Model file for the job. Use its own axes, mm. Face numbers are marked on the shaded views. A direction names the side the tool comes from. Round coordinates to 2 decimals unless told otherwise and drop trailing zeros. Write each loop counter-clockwise with the first axis right and the second up, starting at its lowest first coordinate (ties: lowest second). Pieces come first, ordered by that corner, then holes. Notation, with made-up numbers: (-23, 60) - (-19, 60) arc R11 cw to (-19, 67) - close; hole circle Ø7 at (79, 35). An arc over 180 degrees is marked (long way). One line per item, written item: value.
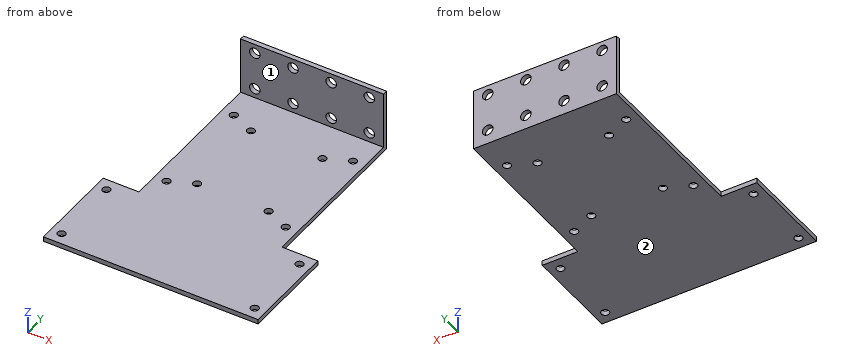
from build123d import *

# Parameters (mm, degrees)
F0_W     = 90
F0_H     = 110
F1_DEPTH = 26
F2_W     = 108
F2_H     = 24
F3_DEPTH = 90.001
F5_D     = 4.4
F6_W     = 15
F6_H     = 70
F7_DEPTH = 26.001
F9_D     = 3.3


with BuildPart() as f1:
    # F0 (on Top) → F1 (new body)
    with BuildSketch(Plane.XY):
        Rectangle(F0_W, F0_H)
    extrude(amount=F1_DEPTH)

    # F2 (on face) → F3 (cut, through all)
    with BuildSketch(Plane.YZ.offset(45)):
        with Locations((-1, 14)):
            Rectangle(F2_W, F2_H)
    extrude(amount=-F3_DEPTH, mode=Mode.SUBTRACT)

    # F5 (through all)
    with Locations(Plane(origin=(0, 55, 0), x_dir=(-1, 0, 0), z_dir=(0, 1, 0))):
        with Locations((-8, 22), (8, 22), (8, 6), (-8, 6), (-24, 22), (24, 22), (24, 6), (-24, 6)):
            Hole(F5_D / 2)

    # F6 (on face) → F7 (cut, through all)
    with BuildSketch(Plane(origin=(0, 0, 0), x_dir=(1, 0, 0), z_dir=(0, 0, -1))):
        with Locations((-37.5, -20)):
            Rectangle(F6_W, F6_H)
        with Locations((37.5, -20)):
            Rectangle(F6_W, F6_H)
    extrude(amount=-F7_DEPTH, mode=Mode.SUBTRACT)

    # F9 (through all)
    with Locations(Plane.XY.offset(2)):
        with Locations((25, 40.5), (15, 36), (-15, 36), (-25, 40.5), (-25, -4.5), (-15, 0), (15, 0), (25, -4.5), (40.5, -20), (40.5, -50), (-40.5, -50), (-40.5, -20)):
            Hole(F9_D / 2)


solid = f1.part
1. Wall check: probe 1 along Z at (x, y) = (8, 53.8); probe 2 along Z at (x, y) = (19, -42.5); probe 3 along Y at (x, z) = (10, 23.75). Give the ranges that are in metal, low to high. Write a range as [from, to].
Report:
probe 1: [0, 3.8], [8.2, 19.8], [24.2, 26]
probe 2: [0, 2]
probe 3: [53, 55]
2. Band-saw the part on A-A on y = 36. Write the cut outline in (x, z).
Report:
outline: (-30, 0) - (-16.65, 0) - (-16.65, 2) - (-30, 2) - close; (-13.35, 0) - (13.35, 0) - (13.35, 2) - (-13.35, 2) - close; (16.65, 0) - (30, 0) - (30, 2) - (16.65, 2) - close
3. Band-saw the part on B-B on x = 15. Write the cut outline in (y, z), plus the area to 3 significant figures.
Report:
outline: (-55, 0) - (-1.65, 0) - (-1.65, 2) - (-55, 2) - close; (1.65, 0) - (34.35, 0) - (34.35, 2) - (1.65, 2) - close; (37.65, 0) - (55, 0) - (55, 26) - (53, 26) - (53, 2) - (37.65, 2) - close
area: 255 mm²
4. Band-saw the part on D-D on x = -40.5. Write the cut outline in (y, z), plus the area to 3 significant figures.
Report:
outline: (-55, 0) - (-51.65, 0) - (-51.65, 2) - (-55, 2) - close; (-48.35, 0) - (-21.65, 0) - (-21.65, 2) - (-48.35, 2) - close; (-18.35, 0) - (-15, 0) - (-15, 2) - (-18.35, 2) - close
area: 66.8 mm²
5. Tool access for the marked faces 1 and 2: list every direction of +Z, -Z, +X, -X, +Y, -Y with a clear straight run to the whole face (end or side of a thin tool).
Report:
face 1: +Z, +X, -X, -Y
face 2: -Z, +X, -X, +Y, -Y
6. Band-saw the part on C-C on x = -25. Write the cut outline in (y, z).
Report:
outline: (-55, 0) - (-6.15, 0) - (-6.15, 2) - (-55, 2) - close; (-2.85, 0) - (38.85, 0) - (38.85, 2) - (-2.85, 2) - close; (42.15, 0) - (55, 0) - (55, 4.04) - (53, 4.04) - (53, 2) - (42.15, 2) - close; (53, 7.96) - (55, 7.96) - (55, 20.04) - (53, 20.04) - close; (53, 23.96) - (55, 23.96) - (55, 26) - (53, 26) - close
7. Drop flat-ended pins along their axis: pin 1 (2 mm diameter, centred on x = -1.5, z = 7, fed in from -Y); pin 2 (3.5 mm diameter, centred on x = 8, z = 6, fed in from +Y); pin 3 (4.5 mm diameter, centred on x = -25, y = -4.5, fed in from +Z). Give the stop position or say it passes through.
Report:
pin 1: y = 53
pin 2: through
pin 3: z = 2
